Check sheet for the modelled part. Datum: model origin and axes. Units: mm. Face numbers are marked on the shaded views. A direction names the side the tool comes from. Coordinates: 2 decimals unless noted, no trailing zeros. Write each loop counter-clockwise with the first axis right and the second up, starting at its lowest first coordinate (ties: lowest second). Pieces come first, ordered by that corner, then holes. Notation, with made-up numbers: M 40.5,40.5 L 45.5,40.5 A14 cw 45.5,53.5 Z; hole C 15.25,22.5 d8. An arc over 180 degrees is marked long. Answer as CSV lines item,"result". Start each with the question number.
Q1. Sectioned sample at D-D, the plane x = 22. Record the cut outline in (y, z).
Q2. Sectioned sample at B-B, the plane x = 4. Record the cut outline in (y, z), then the cut area to 3 significant figures.
Q3. Mould release check, pull along X, two halves, no side actions. Record for the marked faces 3, 4 and 5: pulls with the +X half, pulls with the -X half, needs draft (parallel to the pull), parting line crosses it, or undercut.
Q4. Sectioned sample at C-C, the plane y = 1. Record the cut outline in (x, z).
Q5. Sectioned sample at A-A, the plane z = -4. Record the cut outline in (x, y).
Q6. Thickness scan on line 1 along Z through (x, y) = (4, 6); line 2 along Z through (x, y) = (21, 7.75); line 3 along Z through (x, y) = (33, 6.5). Record the ranges inside material, lowest first. Write a range as from..to.
Q7. Access from +Z, -Z, +X, -X, +Y, -Y to the whole of each face (thin tool, end or side, straight path). Record for the marked faces 1 and 2.
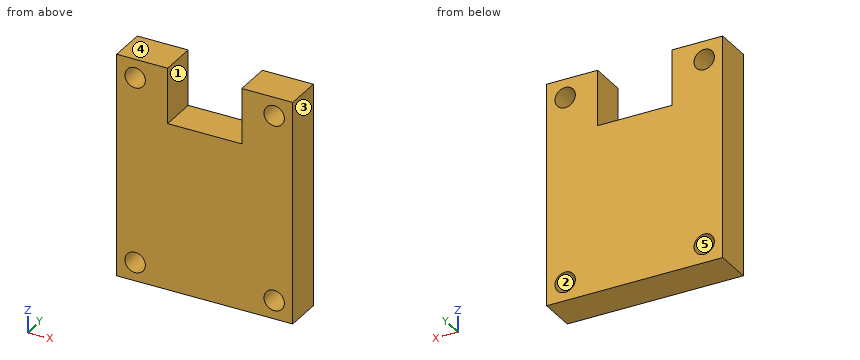
from build123d import *

# Parameters (mm, degrees)
ESQUISSE1_W             = 38
ESQUISSE1_H             = 48
BOSS_EXTRU_1_DEPTH      = 8
ESQUISSE3_R             = 2.2
ENL_V_MAT_EXTRU_1_DEPTH = 8
ENL_V_MAT_EXTRU_2_DEPTH = 8


with BuildPart() as part:
    # Esquisse1 → Boss.-Extru.1 (new body)
    with BuildSketch(Plane(origin=(0, 0, 0), x_dir=(1, 0, 0), z_dir=(0, 1, 0))):
        with Locations((19, 24)):
            Rectangle(ESQUISSE1_W, ESQUISSE1_H)
    extrude(amount=BOSS_EXTRU_1_DEPTH)

    # Esquisse3 → Enlèv. mat.-Extru.1 (cut)
    with BuildSketch(Plane.XZ):
        with Locations((4, -4)):
            Circle(ESQUISSE3_R)
        with Locations((34, -4)):
            Circle(ESQUISSE3_R)
        with Locations((34, -44)):
            Circle(ESQUISSE3_R)
        with Locations((4, -44)):
            Circle(ESQUISSE3_R)
    extrude(amount=-ENL_V_MAT_EXTRU_1_DEPTH, mode=Mode.SUBTRACT)

    # Esquisse5 → Enlèv. mat.-Extru.2 (cut)
    with BuildSketch(Plane(origin=(0, 8, 0), x_dir=(1, 0, 0), z_dir=(0, 1, 0))):
        Polygon((19, 12), (27, 12), (27, 0), (11, 0), (11, 12), align=None)
    extrude(amount=-ENL_V_MAT_EXTRU_2_DEPTH, mode=Mode.SUBTRACT)


solid = part.part
Output:
1,outline,"M 0,-48 L 8,-48 L 8,-12 L 0,-12 Z"
2,outline,"M 0,-48 L 8,-48 L 8,-46.2 L 0,-46.2 Z; M 0,-41.8 L 8,-41.8 L 8,-6.2 L 0,-6.2 Z; M 0,-1.8 L 8,-1.8 L 8,0 L 0,0 Z"
2,area,"314 mm^2"
3,face 3,"pulls with the +X half"
3,face 4,"needs draft"
3,face 5,"undercut"
4,outline,"M 0,-48 L 38,-48 L 38,0 L 27,0 L 27,-12 L 11,-12 L 11,0 L 0,0 Z; hole C 4,-44 d4.4; hole C 4,-4 d4.4; hole C 34,-44 d4.4; hole C 34,-4 d4.4"
5,outline,"M 0,0 L 1.8,0 L 1.8,8 L 0,8 Z; M 6.2,0 L 11,0 L 11,8 L 6.2,8 Z; M 27,0 L 31.8,0 L 31.8,8 L 27,8 Z; M 36.2,0 L 38,0 L 38,8 L 36.2,8 Z"
6,line 1,"z = -48..-46.2, -41.8..-6.2, -1.8..0"
6,line 2,"z = -48..-12"
6,line 3,"z = -48..-45.96, -42.04..-5.96, -2.04..0"
7,face 1,"+Z, +Y, -Y"
7,face 2,"+Y, -Y"
